Source: CAD feature listing. Evaluate the final solid. Frame: model axes, mm. Face numbers are marked on the shaded views. A direction names the side the tool comes from. Give positions to 0.01 mm unless a question says otherwise; leave off trailing zeros. Order: outer loops, then holes, each group sorted by start corner. A loop starts at its lowest first (then second) coordinate and runs counter-clockwise, first axis right, second up. Notation, with made-up numbers: M 84.25,-36 L 106.25,-36 A28 cw 106.25,-11 Z; hole C 81.5,24 d11. An arc over 180 degrees is marked long. Answer as a JSON object with one key per item and string values. Group by question number.
1. Set-up query: the marked faces 1 and 2. Return all of +Z, -Z, +X, -X, +Y, -Y with unobstructed straight access to the full face (end or side cutting, diameter ignored); none if empty.
2. Pull-direction query (X, two-part tool) for the marked faces 3, 4, 5 and 6; classes: +X half, -X half, draft (parallel to the pull), parting line (faces both ways), or undercut.
3. Pin query (flat end, axial travel): P1, Ø1.5, axis at y = 8, z = 18.5, coming from the -X side; P2, Ø12, axis at x = 12.5, y = 3.5, coming from the -Z side; P3, Ø4, axis at y = 11, z = 9, coming from the +X side. Return the tip coordinate at first contact, or that it passes through.
4. Section query D-D (z = 25.5). Output: boundary loops of the cut face in (x, y), plus the area to 3 significant figures.
5. Material intervals for L1, parallel to X at y = -8.5, z = 12; L2, parallel to Z at x = 0, y = -12.5; L3, parallel to Z at x = 14, y = -4, sorted ascending. Write a range as [from, to].
6. Section query A-A (z = 16.5). Output: boundary loops of the cut face in (x, y).
7. Section query C-C (x = 0). Count the separate pieces of the cut face and the enclosed holes in it, plus the area to 3 significant figures.
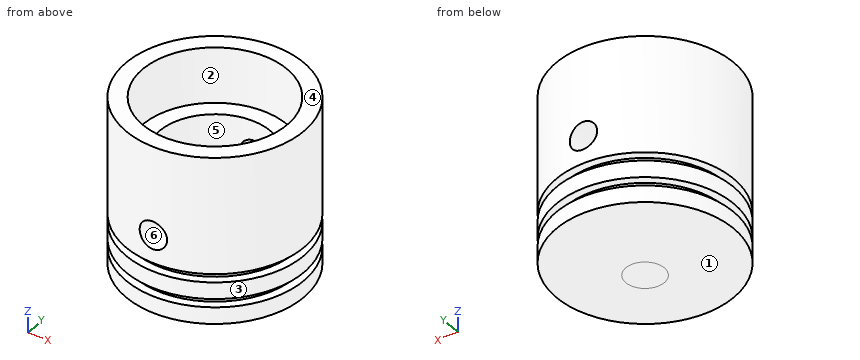
from build123d import *

# Parameters (mm, degrees)
SKETCH3_R          = 2.5
CUT_EXTRUDE1_DEPTH = 40


with BuildPart() as part:
    # Sketch1 → Revolve1 (revolve)
    with BuildSketch(Plane(origin=(0, 0, 0), x_dir=(1, 0, 0), z_dir=(0, 1, 0)), mode=Mode.PRIVATE) as revolve1_sk:
        with BuildLine():
            Line((16, -2.512699454), (3.472963553, -0.30384494))
            ThreePointArc((3.472963553, -0.30384494), (1.743114855, -0.076106038), (0, 0))
            Line((0, 0), (0, -8.512699454))
            Line((0, -8.512699454), (10, -8.512699454))
            Line((10, -8.512699454), (10, -22.512699454))
            Line((10, -22.512699454), (13, -22.512699454))
            Line((13, -22.512699454), (13, -32.512699454))
            Line((13, -32.512699454), (16, -32.512699454))
            Line((16, -32.512699454), (16, -11.512699454))
            Line((16, -11.512699454), (14.5, -11.512699454))
            Line((14.5, -11.512699454), (14.5, -10.012699454))
            Line((14.5, -10.012699454), (16, -10.012699454))
            Line((16, -10.012699454), (16, -7.012699454))
            Line((16, -7.012699454), (14.5, -7.012699454))
            Line((14.5, -7.012699454), (14.5, -5.512699454))
            Line((14.5, -5.512699454), (16, -5.512699454))
            Line((16, -5.512699454), (16, -2.512699454))
        make_face()
    revolve(revolve1_sk.sketch.rotate(Axis((0, 0, 0), (0, 0, 1)), 180), axis=Axis((0, 0, 0), (0, 0, 1)))

    # Sketch3 → Cut-Extrude1 (cut, symmetric)
    with BuildSketch(Plane(origin=(0, 0, 0), x_dir=(0, 0, -1), z_dir=(0, 1, 0))):
        with Locations(Location((-16.512699454, 0, 0), (0, 0, 180))):
            Circle(SKETCH3_R)
    extrude(amount=CUT_EXTRUDE1_DEPTH, both=True, mode=Mode.SUBTRACT)


solid = part.part
Answer sheet:
{
 "1": {"face 1": "-Z", "face 2": "+Z"},
 "2": {"face 3": "parting line", "face 4": "draft", "face 5": "undercut", "face 6": "undercut"},
 "3": {"P1": "x = -14.26", "P2": "z = 0.92", "P3": "x = 13.23"},
 "4": {"outline": "C 0,0 d32; hole C 0,0 d26", "area": "273 mm^2"},
 "5": {"L1": "[-13.56, -5.27], [5.27, 13.56]", "L2": "[1.9, 14.01], [19.01, 22.51]", "L3": "[2.26, 5.51], [7.01, 10.01], [11.51, 32.51]"},
 "6": {"outline": "M -2.5,-15.8 L -2.5,-9.68 A10 cw -2.5,9.68 L -2.5,15.8 A16 ccw Z; M 2.5,-15.8 A16 ccw 2.5,15.8 L 2.5,9.68 A10 cw 2.5,-9.68 Z"},
 "7": {"separate pieces": "3", "enclosed holes": "0", "area": "395 mm^2"}
}
